from build123d import *

# Parameters (mm, degrees)
SKETCH1_W           = 120
SKETCH1_H           = 45.3
BOSS_EXTRUDE1_DEPTH = 6
SKETCH2_W           = 10
SKETCH2_H           = 6
SKETCH2_W_2         = 20
SKETCH2_W_3         = 6
SKETCH2_H_2         = 20
CUT_EXTRUDE1_DEPTH  = 6


with BuildPart() as part:
    # Sketch1 → Boss-Extrude1 (new body)
    with BuildSketch(Plane.XY):
        with Locations((60, -22.65)):
            Rectangle(SKETCH1_W, SKETCH1_H)
    extrude(amount=BOSS_EXTRUDE1_DEPTH)

    # Sketch2 → Cut-Extrude1 (cut)
    with BuildSketch(Plane.XY.offset(6)):
        with Locations((5, -3)):
            Rectangle(SKETCH2_W, SKETCH2_H)
        with Locations((40, -3)):
            Rectangle(SKETCH2_W_2, SKETCH2_H)
        with Locations((80, -3)):
            Rectangle(SKETCH2_W_2, SKETCH2_H)
        with Locations((115, -3)):
            Rectangle(SKETCH2_W, SKETCH2_H)
        with Locations((117, -25.3)):
            Rectangle(SKETCH2_W_3, SKETCH2_H_2)
        with Locations((3, -25.3)):
            Rectangle(SKETCH2_W_3, SKETCH2_H_2)
    extrude(amount=-CUT_EXTRUDE1_DEPTH, mode=Mode.SUBTRACT)


solid = part.part
Work out the finished part from the listing and answer in its coordinate system (mm). A direction names the side the tool comes from. Give positions to 0.01 mm unless a question says otherwise; leave off trailing zeros. Loops run counter-clockwise (first coordinate to the right, second up) from the corner with the lowest first, then second, coordinate; pieces in that order, holes last. Notation, with made-up numbers: (17, 72) - (31, 72) arc R13 ccw to (31, 77) - close; hole circle Ø11 at (75.25, 56). An arc over 180 degrees is marked (long way). Answer in a Markdown table with one row per item. Add a question column.
Q1. A tool of negligible diameter and unlimited length cuts with its end or side. For faces 4 (the flat face through (6, -25, 3)), 5 (the flat face through (110, -3, 3)), 6 (the flat face through (117, -15.3, 3)), 7 (the flat face through (5, -6, 3)), 8 (the flat face through (80, -6, 3)), from which of +Z, -Z, +X, -X, +Y, -Y can it reach the whole face along a straight path? Write none if from no direction.
Q2. The part is cut by section A-A (z = 4.3). Determine the outline of the cut face in (x, y).
Q3. Consider line 1 along X through (y, z) = (-2, 1.4); line 2 along Y through (x, z) = (41, 5.05); line 3 along X through (y, z) = (-33.5, 0.7). Determine where each line is inside the solid, lowest interval first.
Q4. Determine the mould class of faces 1 (the flat face through (114, -25, 3)), 2 (the flat face through (40, -6, 3)), 3 (the flat face through (3, -15.3, 3)) for opening direction X: released by +X, released by -X, zero draft, split by the parting line, or undercut.
Q5. The part is cut by section B-B (x = 73). Determine the outline of the cut face in (y, z).
Q6. Each of these flat-tipped pins is pushed along its axis until it touches: P1, Ø3, axis at x = 43.5, z = 2, coming from the +Y side; P2, Ø2, axis at y = -21, z = 4, coming from the -X side; P3, Ø1.8, axis at y = -4, z = 1.5, coming from the +X side. Where does it stop, or does it pass through?
Q7. The part is cut by section C-C (y = -31). Determine the outline of the cut face in (x, z).
Solution:
| question | item | result |
|---|---|---|
| 1 | face 4 | +Z, -Z, -X |
| 1 | face 5 | +Z, -Z, +X, +Y |
| 1 | face 6 | +Z, -Z, +X |
| 1 | face 7 | +Z, -Z, -X, +Y |
| 1 | face 8 | +Z, -Z, +Y |
| 2 | outline | (0, -45.3) - (120, -45.3) - (120, -35.3) - (114, -35.3) - (114, -15.3) - (120, -15.3) - (120, -6) - (110, -6) - (110, 0) - (90, 0) - (90, -6) - (70, -6) - (70, 0) - (50, 0) - (50, -6) - (30, -6) - (30, 0) - (10, 0) - (10, -6) - (0, -6) - (0, -15.3) - (6, -15.3) - (6, -35.3) - (0, -35.3) - close |
| 3 | line 1 | x = 10 to 30, 50 to 70, 90 to 110 |
| 3 | line 2 | y = -45.3 to -6 |
| 3 | line 3 | x = 6 to 114 |
| 4 | face 1 | released by +X |
| 4 | face 2 | undercut |
| 4 | face 3 | zero draft |
| 5 | outline | (-45.3, 0) - (-6, 0) - (-6, 6) - (-45.3, 6) - close |
| 6 | P1 | stops at y = -6 |
| 6 | P2 | stops at x = 6 |
| 6 | P3 | stops at x = 110 |
| 7 | outline | (6, 0) - (114, 0) - (114, 6) - (6, 6) - close |
